Geometry check sheet. Reference: the model listing, model coordinates, mm. A direction names the side the tool comes from. Round coordinates to 2 decimals unless told otherwise and drop trailing zeros. Order: outer loops, then holes, each group sorted by start corner. A loop starts at its lowest first (then second) coordinate and runs counter-clockwise, first axis right, second up. Notation, with made-up numbers: (73.5, 32) - (95.5, 32) arc R24 cw to (95.5, 52) - close; hole circle Ø2 at (-4.5, 45). An arc over 180 degrees is marked (long way). One line per question, with ' | ' between items. Start each with the question number.
Q1. Sectioned sample at B-B, the plane y = 202. Enter the section's corners in (x, z).
Q2. Tool access check on faces 1 (the face through (-397.465, 88.235, 92.614)), 2 (the face through (375, 30, -130)), 3 (the face through (-5, 293, -82.5)). Record the directions out of +Z, -Z, +X, -X, +Y, -Y that give a thin tool (end or side, any length) a straight path to the whole face; none if there is none.
Q3. Sectioned sample at D-D, the plane y = 132. Enter the section's corners in (x, z).
Q4. Sectioned sample at A-A, the plane z = 68.5. Enter the section's corners in (x, y), then the cut area to 3 significant figures.
Q5. Sectioned sample at C-C, the plane x = -37. Enter the section's corners in (y, z), then the cut area to 4 significant figures.
Q6. Material ranges on line 1 along Z through (x, y) = (-138.5, 274); line 2 along X through (y, z) = (141.5, -82.5); line 3 along Y through (x, z) = (-133, 74), recorded low to high.
Q7. Mould release check, pull along Z, two halves, no side actions. Record for faces 4 (the face through (-378, 28, 135)), 5 (the face through (377.815, 187.313, -108.383)), 6 (the face through (-5, 290, 77.5)): +Z half, -Z half, draft (parallel to the pull), parting line (faces both ways), or undercut.
Q8. Gauge pin test, flat ends, axial feed: P1, Ø13.5, axis at x = -32, y = 303, coming from the -Z side; P2, Ø1.5, axis at x = 150, z = 80, coming from the -Y side; P3, Ø5, axis at x = 48.5, z = 43, coming from the -Y side. Record the tip position at first contact, or that the pin passes through.
```python
from build123d import *

# Parameters (mm, degrees)
CROQUIS1_W              = 800
CROQUIS1_H              = 270
SALIENTE_EXTRUIR1_DEPTH = 315
CROQUIS2_W              = 710
CROQUIS2_H              = 52.5
CORTAR_EXTRUIR2_DEPTH   = 315
CORTAR_EXTRUIR6_DEPTH   = 800
CROQUIS8_W              = 710
CROQUIS8_H              = 270
CORTAR_EXTRUIR7_DEPTH   = 200
VACIADO5_START          = -395
VACIADO5_OUTLINE_W      = 40
VACIADO5_OUTLINE_H      = 155
VACIADO5_DEPTH          = 790
VACIADO5_2_DEPTH        = 40
VACIADO5_START_2        = 355
VACIADO5_3_DEPTH        = 40
CORTAR_EXTRUIR8_DEPTH   = 800


# Read off the part's stored shape, not the designer's step: Vaciado5
with BuildPart() as part:
    # Croquis1 → Saliente-Extruir1 (new body)
    with BuildSketch(Plane(origin=(0, 0, 0), x_dir=(1, 0, 0), z_dir=(0, 1, 0))):
        Rectangle(CROQUIS1_W, CROQUIS1_H)
    extrude(amount=SALIENTE_EXTRUIR1_DEPTH)

    # Croquis2 → Cortar-Extruir2 (cut)
    with BuildSketch(Plane(origin=(0, 315, 0), x_dir=(1, 0, 0), z_dir=(0, 1, 0))):
        with Locations((0, 108.75)):
            Rectangle(CROQUIS2_W, CROQUIS2_H)
        with Locations((0, -108.75)):
            Rectangle(CROQUIS2_W, CROQUIS2_H)
    extrude(amount=-CORTAR_EXTRUIR2_DEPTH, mode=Mode.SUBTRACT)

    # Croquis4 → Cortar-Extruir6 (cut)
    with BuildSketch(Plane(origin=(400, 0, 0), x_dir=(0, 0, -1), z_dir=(1, 0, 0))):
        Polygon((135, 315), (82.5, 315), (135, 56), align=None)
        Polygon((-135, 315), (-82.5, 315), (-135, 56), align=None)
    extrude(amount=-CORTAR_EXTRUIR6_DEPTH, mode=Mode.SUBTRACT)

    # Croquis8 → Cortar-Extruir7 (cut)
    with BuildSketch(Plane.XY.offset(82.5)):
        with Locations((0, 135)):
            Rectangle(CROQUIS8_W, CROQUIS8_H)
    extrude(amount=-CORTAR_EXTRUIR7_DEPTH, mode=Mode.SUBTRACT)

    # Vaciado5 outline → Vaciado5 (cut)
    with BuildSketch(Plane.YZ.offset(VACIADO5_START)):
        with Locations((290, 0)):
            Rectangle(VACIADO5_OUTLINE_W, VACIADO5_OUTLINE_H)
    extrude(amount=VACIADO5_DEPTH, mode=Mode.SUBTRACT)

    # Vaciado5 2 outline → Vaciado5 2 (cut)
    with BuildSketch(Plane.YZ.offset(VACIADO5_START)):
        Polygon((5, 130), (5, -130), (55.498344425, -130), (310, -78.411826573), (310, -77.5), (270, -77.5), (270, 77.5), (310, 77.5), (310, 78.411826573), (55.498344425, 130), align=None)
    extrude(amount=VACIADO5_2_DEPTH, mode=Mode.SUBTRACT)

    # Vaciado5 3 outline → Vaciado5 3 (cut)
    with BuildSketch(Plane.YZ.offset(VACIADO5_START_2)):
        Polygon((5, 130), (5, -130), (55.498344425, -130), (310, -78.411826573), (310, -77.5), (270, -77.5), (270, 77.5), (310, 77.5), (310, 78.411826573), (55.498344425, 130), align=None)
    extrude(amount=VACIADO5_3_DEPTH, mode=Mode.SUBTRACT)

    # Croquis9 → Cortar-Extruir8 (cut)
    with BuildSketch(Plane(origin=(400, 0, 0), x_dir=(0, 0, -1), z_dir=(1, 0, 0))):
        Polygon((-102.5, 35), (102.5, 35), (83, 140), (-83, 140), align=None)
        Polygon((-77.5, 172), (77.5, 172), (57.5, 277), (-57.5, 277), align=None)
    extrude(amount=-CORTAR_EXTRUIR8_DEPTH, mode=Mode.SUBTRACT)


solid = part.part
```
Determined:
1) outline: (-400, -105.41) - (-355, -105.41) - (-355, -100.3) - (-395, -100.3) - (-395, -71.79) - (-400, -71.79) - close; (-400, 71.79) - (-395, 71.79) - (-395, 100.3) - (-355, 100.3) - (-355, 105.41) - (-400, 105.41) - close; (355, -105.41) - (400, -105.41) - (400, -71.79) - (395, -71.79) - (395, -100.3) - (355, -100.3) - close; (355, 100.3) - (395, 100.3) - (395, 71.79) - (400, 71.79) - (400, 105.41) - (355, 105.41) - close
2) face 1: +X, -X | face 2: none | face 3: -Z, +Y, -Y
3) outline: (-400, -119.59) - (-355, -119.59) - (-355, -114.49) - (-395, -114.49) - (-395, -84.49) - (-400, -84.49) - close; (-400, 84.49) - (-395, 84.49) - (-395, 114.49) - (-355, 114.49) - (-355, 119.59) - (-400, 119.59) - close; (355, -119.59) - (400, -119.59) - (400, -84.49) - (395, -84.49) - (395, -114.49) - (355, -114.49) - close; (355, 114.49) - (395, 114.49) - (395, 84.49) - (400, 84.49) - (400, 119.59) - (355, 119.59) - close
4) outline: (-400, 0) - (-355, 0) - (-355, 5) - (-395, 5) - (-395, 35) - (-400, 35) - close; (-400, 140) - (-395, 140) - (-395, 172) - (-400, 172) - close; (-400, 219.25) - (-395, 219.25) - (-395, 310) - (395, 310) - (395, 219.25) - (400, 219.25) - (400, 315) - (-400, 315) - close; (355, 0) - (400, 0) - (400, 35) - (395, 35) - (395, 5) - (355, 5) - close; (395, 140) - (400, 140) - (400, 172) - (395, 172) - close | area: 5,980 mm2
5) outline: (270, -82.5) - (315, -82.5) - (315, 82.5) - (270, 82.5) - (270, 77.5) - (310, 77.5) - (310, -77.5) - (270, -77.5) - close | area: 1,225 mm2
6) line 1: z = -82.5 to -77.5, 77.5 to 82.5 | line 2: x = -400 to -395, 395 to 400 | line 3: y = 310 to 315
7) face 4: +Z half | face 5: -Z half | face 6: undercut
8) P1: stops at z = -82.5 | P2: stops at y = 270 | P3: stops at y = 310
